Geometry check sheet. Reference: the model listing, model coordinates, mm. A direction names the side the tool comes from. Round coordinates to 2 decimals unless told otherwise and drop trailing zeros. Order: outer loops, then holes, each group sorted by start corner. A loop starts at its lowest first (then second) coordinate and runs counter-clockwise, first axis right, second up.
(1) Cross-section at C-C on x = 58.5. Enter the section's corners in (y, z).
(2) Cross-section at A-A on y = 8. Enter the section's corners in (x, z), and give its area (3 significant figures).
(3) Gauge pin test, flat ends, axial feed: P1, Ø1.2, axis at x = 57, z = 3, coming from the -Y side; P2, Ø2, axis at x = 64.5, z = 2, coming from the +Y side. Record the tip position at first contact, or that the pin passes through.
(4) Cross-section at D-D on x = 80. Enter the section's corners in (y, z).
(5) Cross-section at B-B on z = 2.45. Enter the section's corners in (x, y), and give its area (3 significant figures).
(6) Set-up check for faces 1 (the face through (58, 3, 2)), 2 (the face through (10, -9.5, 2)), 3 (the face through (77.98, -3.58, 1.97)): record each of +Z, -Z, +X, -X, +Y, -Y from which the full face is reachable in a straight line by a thin tool's end or side.
(7) Thickness scan on L1, parallel to X at y = 4.5, z = 0.85; L2, parallel to Y at x = 57, z = 2.45; L3, parallel to X at y = -6.25, z = 0.9. Record the ranges inside material, lowest first.
from build123d import *

# Parameters (mm, degrees)
F1_DEPTH = 4


with BuildPart() as f1:
    # F0 (on Top) → F1 (new body)
    with BuildSketch(Plane.XY):
        with BuildLine():
            Line((0, 9.5), (0, 0))
            Line((0, 0), (0, -9.5))
            Line((0, -9.5), (19.44, -9.5))
            ThreePointArc((19.44, -9.5), (26.656878, -8.435678), (33.25927, -5.333333))
            ThreePointArc((33.25927, -5.333333), (36.956609, -3.59602), (40.998061, -3))
            Line((40.998061, -3), (73.998061, -3))
            ThreePointArc((73.998061, -3), (78.039513, -3.596021), (81.736852, -5.333333))
            ThreePointArc((81.736852, -5.333333), (88.3411, -8.436238), (95.56, -9.5))
            Line((95.56, -9.5), (115, -9.5))
            Line((115, -9.5), (115, 0))
            Line((115, 0), (115, 9.5))
            Line((115, 9.5), (95.56, 9.5))
            ThreePointArc((95.56, 9.5), (88.3411, 8.436238), (81.736852, 5.333333))
            ThreePointArc((81.736852, 5.333333), (78.039513, 3.596021), (73.998061, 3))
            Line((73.998061, 3), (40.998061, 3))
            ThreePointArc((40.998061, 3), (36.956609, 3.59602), (33.25927, 5.333333))
            ThreePointArc((33.25927, 5.333333), (26.656878, 8.435678), (19.44, 9.5))
            Line((19.44, 9.5), (0, 9.5))
        make_face()
    extrude(amount=F1_DEPTH)


solid = f1.part
Found:
1. outline: (-3, 0) - (3, 0) - (3, 4) - (-3, 4) - close
2. outline: (0, 0) - (27.97, 0) - (27.97, 4) - (0, 4) - close; (87.03, 0) - (115, 0) - (115, 4) - (87.03, 4) - close
2. area: 224 mm2
3. P1: stops at y = -3
3. P2: stops at y = 3
4. outline: (-4.35, 0) - (4.35, 0) - (4.35, 4) - (-4.35, 4) - close
5. outline: (0, -9.5) - (19.44, -9.5) arc R25 ccw to (33.26, -5.33) arc R14 cw to (41, -3) - (74, -3) arc R14 cw to (81.74, -5.33) arc R25 ccw to (95.56, -9.5) - (115, -9.5) - (115, 9.5) - (95.56, 9.5) arc R25 ccw to (81.74, 5.33) arc R14 cw to (74, 3) - (41, 3) arc R14 cw to (33.26, 5.33) arc R25 ccw to (19.44, 9.5) - (0, 9.5) - close
5. area: 1,500 mm2
6. face 1: +Z, -Z, +Y
6. face 2: +Z, -Z, +X, -X, -Y
6. face 3: +Z, -Z, -Y
7. L1: x = 0 to 34.69, 80.3 to 115
7. L2: y = -3 to 3
7. L3: x = 0 to 31.77, 83.23 to 115
